Check sheet for the modelled part. Datum: model origin and axes. Units: mm. A direction names the side the tool comes from. Coordinates: 2 decimals unless noted, no trailing zeros. Loops run counter-clockwise (first coordinate to the right, second up) from the corner with the lowest first, then second, coordinate; pieces in that order, holes last. Notation, with made-up numbers: M 62.5,-29 L 92.5,-29 A24 cw 92.5,-3 Z; hole C 64.5,-29 d11. An arc over 180 degrees is marked long. Write each question's results on one line, items separated by ' | '. Start each with the question number.
from build123d import *

# Parameters (mm, degrees)
BOSS_EXTRUDE2_DEPTH                          = 2
F_3_2_3_2_DIAMETER_HOLE3_D                   = 3.2
CSK_FOR_M3_FLAT_COUNTERSUNK_HEAD_SCR_2_COUNT = 2
CSK_FOR_M3_FLAT_COUNTERSUNK_HEAD_SCR_2_PITCH = 76
CSK_FOR_M3_FLAT_COUNTERSUNK_HEAD_SCR_3_COUNT = 2
CSK_FOR_M3_FLAT_COUNTERSUNK_HEAD_SCR_3_PITCH = 107.48023074
CSK_FOR_M3_FLAT_COUNTERSUNK_HEAD_SCR_4_COUNT = 2
CSK_FOR_M3_FLAT_COUNTERSUNK_HEAD_SCR_4_PITCH = 76
F_2_2_2_2_DIAMETER_HOLE1_D                   = 2.2
FILLET1_R                                    = 3
FILLET2_R                                    = 1


with BuildPart() as part:
    # Sketch2 → Boss-Extrude2 (new body)
    with BuildSketch(Plane.ZY.offset(51.493641502)):
        Polygon((0.93465612, 3.45185693), (7.43465612, 3.45185693), (7.43465612, 86.45185693), (0.93465612, 86.45185693), (0.93465612, 92.95185693), (-82.06534388, 92.95185693), (-82.06534388, 86.45185693), (-88.56534388, 86.45185693), (-88.56534388, 3.45185693), (-82.06534388, 3.45185693), (-82.06534388, -3.04814307), (0.93465612, -3.04814307), align=None)
        Polygon((-82.06534388, 73.45185693), (-82.06534388, 16.45185693), (-69.06534388, 3.45185693), (-12.06534388, 3.45185693), (0.93465612, 16.45185693), (0.93465612, 73.45185693), (-12.06534388, 86.45185693), (-69.06534388, 86.45185693), align=None, mode=Mode.SUBTRACT)
    extrude(amount=BOSS_EXTRUDE2_DEPTH)

    # Ø3.2 (3.2) Diameter Hole3 (through all)
    with Locations(Plane.ZY.offset(53.493641502)):
        with Locations((-74.06534388, 0.20185693), (-85.31534388, 11.45185693), (-85.31534388, 78.45185693), (-74.06534388, 89.70185693), (-7.06534388, 89.70185693), (4.18465612, 78.45185693), (4.18465612, 11.45185693), (-7.06534388, 0.20185693)):
            Hole(F_3_2_3_2_DIAMETER_HOLE3_D / 2)

    # Sketch24 → CSK for M3 Flat Countersunk Head Screw5 (revolve, cut)
    with BuildSketch(Plane(origin=(-53.493641502, 6.95185693, -78.56534388), x_dir=(0, 0, 1), z_dir=(0, 1, 0))):
        Polygon((0, 0), (0, 2), (1.6, 2), (1.6, 1.65), (3.25, 0), align=None)
    csk_for_m3_flat_countersunk_head_screw5 = revolve(axis=Axis((-59.843641502, 6.95185693, -78.56534388), (1, 0, 0)), mode=Mode.SUBTRACT)

    # CSK for M3 Flat Countersunk Head Scr 2: CSK for M3 Flat Countersunk Head Screw5 ×2
    with Locations(*[(0, i * CSK_FOR_M3_FLAT_COUNTERSUNK_HEAD_SCR_2_PITCH, 0) for i in range(1, CSK_FOR_M3_FLAT_COUNTERSUNK_HEAD_SCR_2_COUNT)]):
        add(csk_for_m3_flat_countersunk_head_screw5, mode=Mode.SUBTRACT)

    # CSK for M3 Flat Countersunk Head Scr 3: CSK for M3 Flat Countersunk Head Screw5 ×2
    with Locations(*[Vector(0, 0.7071067811865478, 0.7071067811865472) * (i * CSK_FOR_M3_FLAT_COUNTERSUNK_HEAD_SCR_3_PITCH) for i in range(1, CSK_FOR_M3_FLAT_COUNTERSUNK_HEAD_SCR_3_COUNT)]):
        add(csk_for_m3_flat_countersunk_head_screw5, mode=Mode.SUBTRACT)

    # CSK for M3 Flat Countersunk Head Scr 4: CSK for M3 Flat Countersunk Head Screw5 ×2
    with Locations(*[(0, 0, i * CSK_FOR_M3_FLAT_COUNTERSUNK_HEAD_SCR_4_PITCH) for i in range(1, CSK_FOR_M3_FLAT_COUNTERSUNK_HEAD_SCR_4_COUNT)]):
        add(csk_for_m3_flat_countersunk_head_screw5, mode=Mode.SUBTRACT)

    # Ø2.2 (2.2) Diameter Hole1 (through all)
    with Locations(Plane(origin=(-53.493641502, 88.95185693, -65.56534388), x_dir=(0, 0, -1), z_dir=(-1, 0, 0))):
        with Locations((0, 0), (-50, 0), (0, 88), (-50, 88)):
            Hole(F_2_2_2_2_DIAMETER_HOLE1_D / 2)

    # Fillet1
    fillet1_edges = [part.edges().sort_by_distance(p)[0] for p in [
        (-52.493641502, 86.45185693, -69.06534388),
        (-52.493641502, 73.45185693, -82.06534388),
        (-52.493641502, 16.45185693, -82.06534388),
        (-52.493641502, 3.45185693, -69.06534388),
        (-52.493641502, 3.45185693, -12.06534388),
        (-52.493641502, 16.45185693, 0.93465612),
        (-52.493641502, 73.45185693, 0.93465612),
        (-52.493641502, 86.45185693, -12.06534388),
    ]]
    fillet(fillet1_edges, radius=FILLET1_R)

    # Fillet2
    fillet2_edges = [part.edges().sort_by_distance(p)[0] for p in [
        (-52.493641502, 3.45185693, -82.06534388),
        (-52.493641502, 86.45185693, -82.06534388),
        (-52.493641502, 86.45185693, 0.93465612),
        (-52.493641502, 3.45185693, 0.93465612),
    ]]
    fillet(fillet2_edges, radius=FILLET2_R)


solid = part.part
Item 1: Thickness scan on line 1 (Z direction, x = -52.3, y = 28); line 2 (Y direction, x = -53.1, z = -15); line 3 (Y direction, x = -52.5, z = -79.5). Record the ranges inside material, lowest first.
Item 2: Section check A-A (y = 26). Record the cut outline in (x, z), plus the area to 3 significant figures.
Item 3: Depth check by flat-ended pin: P1, Ø0.6, axis at x = -52, z = -85, coming from the -Y side; P2, Ø0.6, axis at x = -52.5, y = 1, coming from the +Z side. Enter the tip coordinate at first touch or a pass-through.
Item 4: Section check C-C (x = -53.05). State how many separate pieces and enclosed holes the cut face has, plus the area to 3 significant figures.
Item 5: Tool access check on faces 1 (the face through (-51.95, 7.99, -3.92)), 2 (the face through (-52.48, 79.873, -5.487)). Record the directions out of +Z, -Z, +X, -X, +Y, -Y that give a thin tool (end or side, any length) a straight path to the whole face; none if there is none.
Item 6: Section check B-B (z = -61.5). Record the cut outline in (x, y), plus the area to 3 significant figures.
Item 7: Release check for a two-part mould opening along Z. For faces 3 (the face through (-52, 91, -8)), 4 (the face through (-53.494, 3, -37)) record: +Z half, -Z half, draft (parallel to the pull), parting line (faces both ways), or undercut.
Computed values:
1) line 1: z = -88.57 to -82.07, 0.93 to 7.43 | line 2: y = -3.05 to 0.01, 1.9 to 3.45, 86.45 to 88.01, 89.9 to 92.95 | line 3: y = -3.05 to 4.9, 9.01 to 13.89, 76.02 to 80.9, 85.01 to 92.95
2) outline: M -53.49,-88.57 L -51.49,-88.57 L -51.49,-82.07 L -53.49,-82.07 Z; M -53.49,0.93 L -51.49,0.93 L -51.49,7.43 L -53.49,7.43 Z | area: 26.0 mm²
3) P1: stops at y = 3.45 | P2: stops at z = 0.93
4) separate pieces: 1 | enclosed holes: 17 | area: 2,320 mm²
5) face 1: -X | face 2: +X, -X
6) outline: M -53.49,-3.05 L -51.49,-3.05 L -51.49,3.45 L -53.49,3.45 Z; M -53.49,86.45 L -51.49,86.45 L -51.49,92.95 L -53.49,92.95 Z | area: 26.0 mm²
7) face 3: undercut | face 4: draft
